from build123d import *

# Parameters (mm, degrees)
SKETCH1_W           = 14
SKETCH1_H           = 18
BOSS_EXTRUDE1_DEPTH = 1.6
BOSS_EXTRUDE2_START = -2
SKETCH2_W           = 14
SKETCH2_H           = 6
BOSS_EXTRUDE2_DEPTH = 6
SKETCH3_R           = 1.55
CUT_EXTRUDE1_DEPTH  = 18.029386366


with BuildPart() as part:
    # Sketch1 → Boss-Extrude1 (new body)
    with BuildSketch(Plane.XY):
        Rectangle(SKETCH1_W, SKETCH1_H)
    extrude(amount=BOSS_EXTRUDE1_DEPTH)

    # Sketch2 → Boss-Extrude2 (add)
    with BuildSketch(Plane.XY.offset(1.6).offset(BOSS_EXTRUDE2_START)):
        with Locations((0, 12)):
            Rectangle(SKETCH2_W, SKETCH2_H)
    extrude(amount=BOSS_EXTRUDE2_DEPTH)

    # Sketch3 → Cut-Extrude1 (cut, through all)
    with BuildSketch(Plane.XY.offset(1.6)):
        with Locations((-3.85, -2.45)):
            Circle(SKETCH3_R)
    extrude(amount=-CUT_EXTRUDE1_DEPTH, mode=Mode.SUBTRACT)


solid = part.part
Check sheet for the modelled part. Datum: model origin and axes. Units: mm. A direction names the side the tool comes from. Round coordinates to 2 decimals unless told otherwise and drop trailing zeros. Order: outer loops, then holes, each group sorted by start corner. A loop starts at its lowest first (then second) coordinate and runs counter-clockwise, first axis right, second up.
(1) Cross-section at D-D, the plane z = 3.3. Enter the section's corners in (x, y), and give its area (3 significant figures).
(2) Go/stop test with flat-tipped pins: P1, Ø2.5, axis at x = -3.85, y = -2.45, coming from the +Z side; P2, Ø4, axis at x = 1.5, y = 0.5, coming from the -Z side; P3, Ø7, axis at x = 1.5, y = 3, coming from the +Z side; P4, Ø3, axis at x = -1, z = 4, coming from the -Y side. Record where each tip stops, or that it passes through.
(3) Cross-section at B-B, the plane y = -2.45. Enter the section's corners in (x, z).
(4) Draft check along X on faces 3 (the flat face through (0, 0, 0)), 4 (the cylindrical face through (-2.372, -1.984, 0.811)), 5 (the flat face through (-7, 8, 1)). Enter one of: pulls with the +X half, pulls with the -X half, needs draft (parallel to the pull), parting line crosses it, or undercut.
(5) Cross-section at C-C, the plane x = -0.25. Enter the section's corners in (y, z), and give its area (3 significant figures).
(6) Access from +Z, -Z, +X, -X, +Y, -Y to the whole of each face (thin tool, end or side, straight path). Record for faces 1 (the flat face through (0, 15, 3)), 2 (the flat face through (0, 0, 1.6)).
(7) Scan lines: probe 1 along Y at (x, z) = (-3.85, 0.4); probe 2 along Z at (x, y) = (2.75, 5); probe 3 along Y at (x, z) = (0.5, 3.45). Record each from-to range of solid material in increasing order.
(8) Cross-section at A-A, the plane x = -3.85. Enter the section's corners in (y, z), and give its area (3 significant figures).
Check sheet entries:
1. outline: (-7, 9) - (7, 9) - (7, 15) - (-7, 15) - close
1. area: 84.0 mm2
2. P1: passes through
2. P2: stops at z = 0
2. P3: stops at z = 1.6
2. P4: stops at y = 9
3. outline: (-7, 0) - (-5.4, 0) - (-5.4, 1.6) - (-7, 1.6) - close; (-2.3, 0) - (7, 0) - (7, 1.6) - (-2.3, 1.6) - close
4. face 3: needs draft
4. face 4: undercut
4. face 5: pulls with the -X half
5. outline: (-9, 0) - (9, 0) - (9, -0.4) - (15, -0.4) - (15, 5.6) - (9, 5.6) - (9, 1.6) - (-9, 1.6) - close
5. area: 64.8 mm2
6. face 1: +Z, -Z, +X, -X, +Y
6. face 2: +Z, +X, -X, -Y
7. probe 1: y = -9 to -4, -0.9 to 15
7. probe 2: z = 0 to 1.6
7. probe 3: y = 9 to 15
8. outline: (-9, 0) - (-4, 0) - (-4, 1.6) - (-9, 1.6) - close; (-0.9, 0) - (9, 0) - (9, -0.4) - (15, -0.4) - (15, 5.6) - (9, 5.6) - (9, 1.6) - (-0.9, 1.6) - close
8. area: 59.8 mm2
